```python
from build123d import *

# Parameters (mm, degrees)
F1_DEPTH = 3.81
F2_R     = 1.27
F3_DEPTH = 10.668
F4_W     = 2.54
F4_H     = 3.81
F5_DEPTH = 0.9906
F7_DEPTH = 25.4


with BuildPart() as f1:
    # F0 (on Front) → F1 (new body)
    with BuildSketch(Plane.XZ):
        with BuildLine():
            Line((0, 2.619967), (0, 0))
            Line((0, 0), (2.54, 0))
            Line((2.54, 0), (2.54, 3.558869))
            ThreePointArc((2.54, 3.558869), (2.581181, 4.341032), (2.704268, 5.114547))
            ThreePointArc((2.704268, 5.114547), (3.530295, 12.330484), (2.704268, 19.546421))
            ThreePointArc((2.704268, 19.546421), (2.581201, 20.259234), (2.54, 20.981419))
            Line((2.54, 20.981419), (2.54, 26.571107))
            Line((2.54, 26.571107), (0, 26.571107))
            Line((0, 26.571107), (0, 21.160008))
            ThreePointArc((0, 21.160008), (0.06165, 20.277308), (0.245405, 19.411748))
            ThreePointArc((0.245405, 19.411748), (1.301239, 11.889988), (0.245405, 4.368227))
            ThreePointArc((0.245405, 4.368227), (0.06165, 3.502667), (0, 2.619967))
        make_face()
    extrude(amount=F1_DEPTH)

    # F2 (on face) → F3 (cut)
    with BuildSketch(Plane(origin=(0, 0, 0), x_dir=(0, -1, 0), z_dir=(-1, 0, 0))):
        with Locations((1.905, 23.865558)):
            Circle(F2_R)
    extrude(amount=-F3_DEPTH, mode=Mode.SUBTRACT)

    # F4 (on face) → F5 (join)
    with BuildSketch(Plane(origin=(0, 0, 0), x_dir=(1, 0, 0), z_dir=(0, 0, -1))):
        with Locations((1.27, 1.905)):
            Rectangle(F4_W, F4_H)
    extrude(amount=F5_DEPTH)

    # F6 (on face) → F7 (cut)
    with BuildSketch(Plane(origin=(0, 0, 0), x_dir=(0, -1, 0), z_dir=(-1, 0, 0))):
        with BuildLine():
            ThreePointArc((3.175, 0.814683), (2.803026, 1.712709), (1.905, 2.084683))
            Line((1.905, 2.084683), (1.905, -0.455317))
            ThreePointArc((1.905, -0.455317), (2.803026, -0.083342), (3.175, 0.814683))
        make_face()
        with BuildLine():
            Line((1.905, -0.455317), (1.905, 2.084683))
            ThreePointArc((1.905, 2.084683), (0.635, 0.814683), (1.905, -0.455317))
        make_face()
    extrude(amount=-F7_DEPTH, mode=Mode.SUBTRACT)


solid = f1.part
```
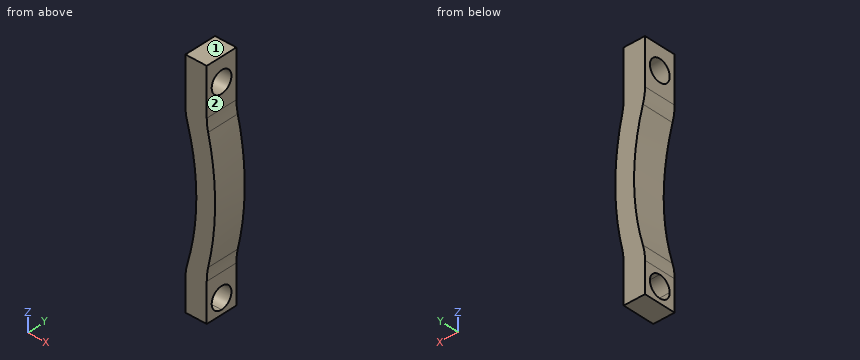
Here's how the part is built. I have some questions about the finished solid (model axes, mm). Face numbers are marked on the shaded views. A direction names the side the tool comes from. Give positions to 0.01 mm unless a question says otherwise; leave off trailing zeros. Loops run counter-clockwise (first coordinate to the right, second up) from the corner with the lowest first, then second, coordinate; pieces in that order, holes last. Notation, with made-up numbers: M -7.5,-27 L 51.5,-27 A29 cw 51.5,-1 Z; hole C -23.75,67.5 d1. An arc over 180 degrees is marked long. Return JSON: item names as keys, results as strings.
Item 1: Please list where these lines run through material, in increasing order: line 1 (Y direction, x = 1.55, z = 0.75); line 2 (Z direction, x = 1.85, y = -1.45); line 3 (Z direction, x = 1.35, y = -2.2).
A:
{"line 1": "y = -3.81 to -3.17, -0.64 to 0", "line 2": "z = -0.99 to -0.37, 2 to 22.68, 25.05 to 26.57", "line 3": "z = -0.99 to -0.42, 2.05 to 22.63, 25.1 to 26.57"}
Item 2: Imagine slicing it at D-D on y = -3.5. List the corners of the cut face in (x, z) for me.
A:
{"outline": "M 0,-0.99 L 2.54,-0.99 L 2.54,3.56 A7.45 cw 2.7,5.11 A31.93 ccw 2.7,19.55 A6.35 cw 2.54,20.98 L 2.54,26.57 L 0,26.57 L 0,21.16 A6.35 ccw 0.25,19.41 A27.32 cw 0.25,4.37 A6.35 ccw 0,2.62 Z"}
Item 3: Imagine slicing it at B-B on z = 23. List the corners of the cut face in (x, y) for me.
A:
{"outline": "M 0,-3.81 L 2.54,-3.81 L 2.54,-2.83 L 0,-2.83 Z; M 0,-0.98 L 2.54,-0.98 L 2.54,0 L 0,0 Z"}
Item 4: Imagine slicing it at C-C on y = -1.55. List the corners of the cut face in (x, z) for me, then the cut area to 3 significant figures.
A:
{"outline": "M 0,-0.99 L 2.54,-0.99 L 2.54,-0.4 L 0,-0.4 Z; M 0,2.03 L 2.54,2.03 L 2.54,3.56 A7.45 cw 2.7,5.11 A31.93 ccw 2.7,19.55 A6.35 cw 2.54,20.98 L 2.54,22.65 L 0,22.65 L 0,21.16 A6.35 ccw 0.25,19.41 A27.32 cw 0.25,4.37 A6.35 ccw 0,2.62 Z; M 0,25.08 L 2.54,25.08 L 2.54,26.57 L 0,26.57 Z", "area": "53.5 mm^2"}
Item 5: Imagine slicing it at A-A on x = 0.7. List the corners of the cut face in (y, z) for me (3 decimals), then the cut area to 3 significant figures.
A:
{"outline": "M -3.81,-0.991 L 0,-0.991 L 0,6.19 L -3.81,6.19 Z; M -3.81,17.59 L 0,17.59 L 0,26.571 L -3.81,26.571 Z; hole M -3.175,0.815 A1.27 ccw long -1.905,2.085 A1.27 ccw Z; hole C -1.905,23.866 d2.54", "area": "51.4 mm^2"}
Item 6: On a 3-axis mill with a long thin cutter (end or side, diameter ignored), from which of +Z, -Z, +X, -X, +Y, -Y can I reach the whole of each face in a straight line? I mean the marked faces 1 and 2. Say none if no direction works.
A:
{"face 1": "+Z, +X, -X, +Y, -Y", "face 2": "+Z, +X, +Y, -Y"}
